Can you work these out from the model? Positions are in its coordinate system, mm. A direction names the side the tool comes from. Give positions to 0.01 mm unless a question says otherwise; leave off trailing zeros. Loops run counter-clockwise (first coordinate to the right, second up) from the corner with the lowest first, then second, coordinate; pieces in that order, holes last. Notation, with made-up numbers: (-39, 68) - (19, 68) arc R35 cw to (19, 101) - close; hole circle Ø9 at (29, 49.25). An arc over 180 degrees is marked (long way). Write item = value, one per line.
from build123d import *

# Parameters (mm, degrees)
SKETCH1_W               = 110
SKETCH1_H               = 77.5
SKETCH1_W_2             = 104
SKETCH1_H_2             = 71.5
BOSS_EXTRUDE1_DEPTH     = 10
SKETCH1_2_W             = 110
SKETCH1_2_H             = 77.5
SKETCH1_2_W_2           = 104
SKETCH1_2_H_2           = 71.5
BOSS_EXTRUDE2_DEPTH     = 3
CUT_EXTRUDE1_REACH      = 136.931
SKETCH3_W               = 15.2
SKETCH3_H               = 6.73
CUT_EXTRUDE2_REACH      = 136.931
SKETCH4_R               = 1.45
SKETCH4_W               = 8.6
SKETCH4_H               = 3.42
CUT_EXTRUDE3_DEPTH      = 135.930537685
CUT_EXTRUDE3_DEPTH_BACK = 135.930537685
SKETCH5_W               = 16.4
SKETCH5_H               = 5
FILLET1_R               = 4
FILLET2_R               = 1


with BuildPart() as part:
    # Sketch1 → Boss-Extrude1 (new body)
    with BuildSketch(Plane(origin=(0, 0, 0), x_dir=(1, 0, 0), z_dir=(0, 1, 0))):
        with Locations((55, 38.75)):
            Rectangle(SKETCH1_W, SKETCH1_H)
        with Locations((55, 38.75)):
            Rectangle(SKETCH1_W_2, SKETCH1_H_2, mode=Mode.SUBTRACT)
    extrude(amount=BOSS_EXTRUDE1_DEPTH)

    # Sketch1_2 → Boss-Extrude2 (add)
    # profile 1 of 2: a face of its own
    with BuildSketch(Plane(origin=(0, 0, 0), x_dir=(1, 0, 0), z_dir=(0, 1, 0))):
        with Locations((55, 38.75)):
            Rectangle(SKETCH1_2_W, SKETCH1_2_H)
        with Locations((55, 38.75)):
            Rectangle(SKETCH1_2_W_2, SKETCH1_2_H_2, mode=Mode.SUBTRACT)
    # profile 2 of 2: a face of its own
    with BuildSketch(Plane(origin=(0, 0, 0), x_dir=(1, 0, 0), z_dir=(0, 1, 0))):
        with Locations((55, 38.75)):
            Rectangle(SKETCH1_2_W_2, SKETCH1_2_H_2)
    extrude(amount=-BOSS_EXTRUDE2_DEPTH)

    # Sketch3 → Cut-Extrude1 (cut, up to next)
    with BuildSketch(Plane.ZY, mode=Mode.PRIVATE) as cut_extrude1_sk1:
        with Locations((-23.5, 6.635)):
            Rectangle(SKETCH3_W, SKETCH3_H)
    cut_extrude1_tool1 = extrude(cut_extrude1_sk1.sketch, amount=-CUT_EXTRUDE1_REACH, mode=Mode.PRIVATE) & part.part
    # Sketch3 → Cut-Extrude1 (cut, up to next)
    with BuildSketch(Plane.ZY, mode=Mode.PRIVATE) as cut_extrude1_sk2:
        with Locations((-59.4, 6.635)):
            Rectangle(SKETCH3_W, SKETCH3_H)
    cut_extrude1_tool2 = extrude(cut_extrude1_sk2.sketch, amount=-CUT_EXTRUDE1_REACH, mode=Mode.PRIVATE) & part.part
    # Sketch3 → Cut-Extrude1 (cut, up to next)
    with BuildSketch(Plane.ZY, mode=Mode.PRIVATE) as cut_extrude1_sk3:
        with BuildLine():
            Line((-37.84, 9.38), (-44.840000134, 9.38))
            ThreePointArc((-44.840000134, 9.38), (-46.254213696, 8.794213562), (-46.840000134, 7.38))
            Line((-46.840000134, 7.38), (-46.840000134, 6.18))
            ThreePointArc((-46.840000134, 6.18), (-46.254213696, 4.765786438), (-44.840000134, 4.18))
            Line((-44.840000134, 4.18), (-37.84, 4.18))
            ThreePointArc((-37.84, 4.18), (-36.425786438, 4.765786438), (-35.84, 6.18))
            Line((-35.84, 6.18), (-35.84, 7.38))
            ThreePointArc((-35.84, 7.38), (-36.425786438, 8.794213562), (-37.84, 9.38))
        make_face()
    cut_extrude1_tool3 = extrude(cut_extrude1_sk3.sketch, amount=-CUT_EXTRUDE1_REACH, mode=Mode.PRIVATE) & part.part
    add(cut_extrude1_tool1.solids().sort_by_distance((0, 6.635, -23.5))[0], mode=Mode.SUBTRACT)
    add(cut_extrude1_tool2.solids().sort_by_distance((0, 6.635, -59.4))[0], mode=Mode.SUBTRACT)
    add(cut_extrude1_tool3.solids().sort_by_distance((0, 6.78, -41.34))[0], mode=Mode.SUBTRACT)

    # Sketch4 → Cut-Extrude2 (cut, up to next)
    with BuildSketch(Plane(origin=(0, 0, -77.5), x_dir=(-1, 0, 0), z_dir=(0, 0, -1)), mode=Mode.PRIVATE) as cut_extrude2_sk1:
        with Locations((-13.93, 6.69)):
            Circle(SKETCH4_R)
    cut_extrude2_tool1 = extrude(cut_extrude2_sk1.sketch, amount=-CUT_EXTRUDE2_REACH, mode=Mode.PRIVATE) & part.part
    # Sketch4 → Cut-Extrude2 (cut, up to next)
    with BuildSketch(Plane(origin=(0, 0, -77.5), x_dir=(-1, 0, 0), z_dir=(0, 0, -1)), mode=Mode.PRIVATE) as cut_extrude2_sk2:
        with Locations((-25.34, 7.17)):
            Rectangle(SKETCH4_W, SKETCH4_H)
    cut_extrude2_tool2 = extrude(cut_extrude2_sk2.sketch, amount=-CUT_EXTRUDE2_REACH, mode=Mode.PRIVATE) & part.part
    add(cut_extrude2_tool1.solids().sort_by_distance((13.93, 6.69, -77.5))[0], mode=Mode.SUBTRACT)
    add(cut_extrude2_tool2.solids().sort_by_distance((25.34, 7.17, -77.5))[0], mode=Mode.SUBTRACT)

    # Sketch5 → Cut-Extrude3 (cut, two sides: drawn at the far end of the back side and taken through both)
    with BuildSketch(Plane(origin=(0, 0, 0), x_dir=(1, 0, 0), z_dir=(0, 1, 0)).offset(-CUT_EXTRUDE3_DEPTH_BACK)):
        with Locations((20.2, 12.2)):
            Rectangle(SKETCH5_W, SKETCH5_H)
    extrude(amount=CUT_EXTRUDE3_DEPTH + CUT_EXTRUDE3_DEPTH_BACK, mode=Mode.SUBTRACT)

    # Fillet1
    fillet1_edges = [part.edges().sort_by_distance(p)[0] for p in [
        (0, 3.5, -77.5),
        (110, 3.5, -77.5),
        (110, 3.5, 0),
        (0, 3.5, 0),
    ]]
    fillet(fillet1_edges, radius=FILLET1_R)

    # Fillet2
    fillet2_edges = [part.edges().sort_by_distance(p)[0] for p in [
        (12, -1.5, -9.7),
        (12, -1.5, -14.7),
        (28.4, -1.5, -14.7),
        (28.4, -1.5, -9.7),
    ]]
    fillet(fillet2_edges, radius=FILLET2_R)


solid = part.part
Q1. Imagine slicing it at A-A, the plane z = -41.5. Write out the boundary of the cut face in (x, y).
Output:
outline = (0, -3) - (110, -3) - (110, 10) - (107, 10) - (107, 0) - (3, 0) - (3, 4.18) - (0, 4.18) - close; (0, 9.38) - (3, 9.38) - (3, 10) - (0, 10) - close
Q2. Which directions (+Z, -Z, +X, -X, +Y, -Y) give clear straight access to the entire face, cutting with the end or side of a thin tool? Please do faces 4 (the flat face through (1, 3.27, -24)), 5 (the flat face through (3, 4, -38)), 6 (the flat face through (25, 5.46, -76)).
Output:
face_4 = -X, +Y
face_5 = +Y
face_6 = -Z
Q3. We'd pull the mould along Z, two halves only. Please class faces 1 (the flat face through (28.4, -2, -12)), 2 (the flat face through (54, 4, 0)), 3 (the flat face through (67, 10, -2)): released by +Z, released by -Z, zero draft, split by the parting line, or undercut.
Output:
face_1 = undercut
face_2 = released by +Z
face_3 = zero draft
Q4. I need wall thicknesses on L1, parallel to Y at x = 13.93, z = -75.5; L2, parallel to Z at x = 52.5, y = 5.5; L3, parallel to Z at x = 22, y = -2.5. Which ranges of each line are inside material? Lowest first, please.
Output:
L1 = -3 to 5.24, 8.14 to 10
L2 = -77.5 to -74.5, -3 to 0
L3 = -77.5 to -14.7, -9.7 to 0
Q5. Imagine slicing it at C-C, the plane z = -69.5. Write out the boundary of the cut face in (x, y).
Output:
outline = (0, -3) - (110, -3) - (110, 10) - (107, 10) - (107, 0) - (3, 0) - (3, 10) - (0, 10) - close
Q6. Imagine slicing it at B-B, the plane x = 37.5. Write out the boundary of the cut face in (y, z).
Output:
outline = (-3, -77.5) - (10, -77.5) - (10, -74.5) - (0, -74.5) - (0, -3) - (10, -3) - (10, 0) - (-3, 0) - close
Q7. For pin 1 (1.5 mm diameter, centred on x = 1.5, y = 7.5, fed in from +Z); pin 2 (1.5 mm diameter, centred on x = 15.5, z = -39, fed in from +Y); pin 3 (0.9 mm diameter, centred on x = 2, y = 6, fed in from -Z), each with a flat end and sliding along its axis, tell me the tip position at first contact or that it passes through.
Output:
pin_1 = -0.4
pin_2 = 0
pin_3 = -77.19
